Work out the finished part from the listing and answer in its coordinate system (mm). Face numbers are marked on the shaded views. A direction names the side the tool comes from. Give positions to 0.01 mm unless a question says otherwise; leave off trailing zeros. Write each loop counter-clockwise with the first axis right and the second up, starting at its lowest first coordinate (ties: lowest second). Pieces come first, ordered by that corner, then holes. Notation, with made-up numbers: (-23, -25.5) -> (12, -25.5) arc R19 cw to (12, 3.5) -> close; hole circle Ø10 at (85, 62). An arc over 180 degrees is marked (long way). Write item = value, one per line. Start each with the question number.
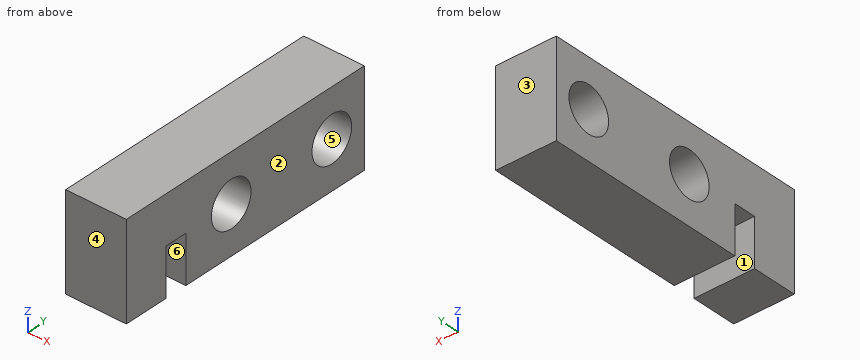
from build123d import *

# Parameters (mm, degrees)
F0_W     = 4
F0_H     = 6.3
F1_DEPTH = 18
F2_W     = 1.5
F2_H     = 3.15
F3_DEPTH = 25
F4_R     = 1.5
F5_DEPTH = 25


with BuildPart() as f1:
    # F0 (on Front) → F1 (new body)
    with BuildSketch(Plane.XZ):
        Rectangle(F0_W, F0_H)
    extrude(amount=F1_DEPTH)

    # F2 (on face) → F3 (cut)
    with BuildSketch(Plane(origin=(-2, 0, 0), x_dir=(0, -1, 0), z_dir=(-1, 0, 0))):
        with Locations((14.25, -1.575)):
            Rectangle(F2_W, F2_H)
    extrude(amount=-F3_DEPTH, mode=Mode.SUBTRACT)

    # F4 (on face) → F5 (cut)
    with BuildSketch(Plane(origin=(-2, 0, 0), x_dir=(0, -1, 0), z_dir=(-1, 0, 0))):
        with Locations((2.45419, 0)):
            Circle(F4_R)
        with Locations((10.06419, 0)):
            Circle(F4_R)
    extrude(amount=-F5_DEPTH, mode=Mode.SUBTRACT)


solid = f1.part
(1) This flat-tipped pin is pushed along its axis until it touches: pin 1 (0.8 mm diameter, centred on x = 0, y = -14.5, fed in from -Z). Where does it stop, or does it pass through?
(2) A cutting plane is placed at C-C, the plane z = 0.5. Write down the section's boundary in (x, y), then the cut area to 3 significant figures.
(3) A cutting plane is placed at B-B, the plane z = -0.75. Write down the section's boundary in (x, y), then the cut area to 3 significant figures.
(4) A cutting plane is placed at A-A, the plane x = 0.2. Write down the section's boundary in (y, z), then the cut area to 3 significant figures.
(5) For the marked faces 5 and 6, determine the directions among +Z, -Z, +X, -X, +Y, -Y from which every point of the face is accessible in a straight line to the end or side of a thin tool.
(6) Find the intervals of material crossed by line 1 along Y through (x, z) = (0.3, -2.5); line 2 along Y through (x, z) = (-0.9, -0.75); line 3 along Y through (x, z) = (0.95, 1), in increasing order.
(7) Determine the mould class of the marked faces 1, 2, 3 and 4 for opening direction Y: pulls with the +Y half, pulls with the -Y half, needs draft (parallel to the pull), parting line crosses it, or undercut.
Results list:
q1.pin_1 = 0
q2.outline = (-2, -18) -> (2, -18) -> (2, -11.48) -> (-2, -11.48) -> close; (-2, -8.65) -> (2, -8.65) -> (2, -3.87) -> (-2, -3.87) -> close; (-2, -1.04) -> (2, -1.04) -> (2, 0) -> (-2, 0) -> close
q2.area = 49.4 mm²
q3.outline = (-2, -18) -> (2, -18) -> (2, -15) -> (-2, -15) -> close; (-2, -13.5) -> (2, -13.5) -> (2, -11.36) -> (-2, -11.36) -> close; (-2, -8.77) -> (2, -8.77) -> (2, -3.75) -> (-2, -3.75) -> close; (-2, -1.16) -> (2, -1.16) -> (2, 0) -> (-2, 0) -> close
q3.area = 45.2 mm²
q4.outline = (-18, -3.15) -> (-15, -3.15) -> (-15, 0) -> (-13.5, 0) -> (-13.5, -3.15) -> (0, -3.15) -> (0, 3.15) -> (-18, 3.15) -> close; hole circle Ø3 at (-10.06, 0); hole circle Ø3 at (-2.45, 0)
q4.area = 94.5 mm²
q5.face_5 = +X, -X
q5.face_6 = -Z, +X, -X
q6.line_1 = -18 to -15, -13.5 to 0
q6.line_2 = -18 to -15, -13.5 to -11.36, -8.77 to -3.75, -1.16 to 0
q6.line_3 = -18 to -11.18, -8.95 to -3.57, -1.34 to 0
q7.face_1 = undercut
q7.face_2 = needs draft
q7.face_3 = pulls with the +Y half
q7.face_4 = pulls with the -Y half
